Source: CAD feature listing. Evaluate the final solid. Frame: model axes, mm. Round coordinates to 2 decimals unless told otherwise and drop trailing zeros. Loops run counter-clockwise (first coordinate to the right, second up) from the corner with the lowest first, then second, coordinate; pieces in that order, holes last. Notation, with made-up numbers: (56, 39) - (91, 39) arc R13 ccw to (91, 45) - close; hole circle Ø11 at (15, 20.5). An arc over 180 degrees is marked (long way). One line per question, with ' | ' between items.
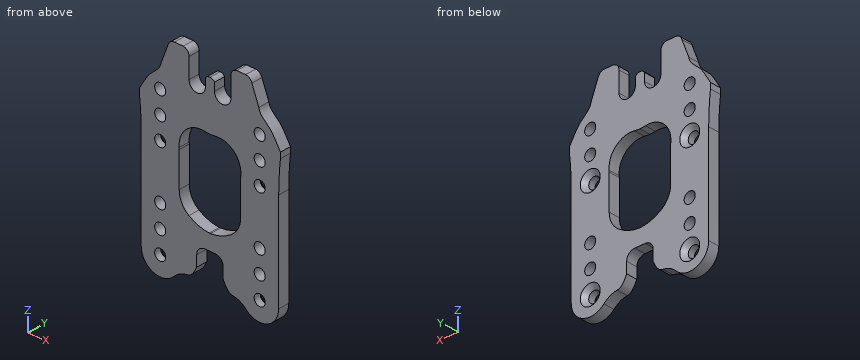
from build123d import *

# Parameters (mm, degrees)
BOSS_EXTRUDE1_DEPTH            = 5
M6_CLEARANCE_HOLE1_D           = 5
M6_CLEARANCE_HOLE1_CSINK_D     = 9
M6_CLEARANCE_HOLE1_CSINK_ANGLE = 90
M6X1_0_TAPPED_HOLE1_D          = 5


with BuildPart() as part:
    # Sketch1 → Boss-Extrude1 (new body)
    with BuildSketch(Plane(origin=(0, 0, 0), x_dir=(1, 0, 0), z_dir=(0, 1, 0))):
        with BuildLine():
            Line((69.154429566, 13.47085249), (69.154429566, 16.004009211))
            ThreePointArc((69.154429566, 16.004009211), (68.568623983, 23.140876552), (68.373161278, 30.2990773))
            Line((68.373161278, 30.2990773), (68.373161278, 48.133269951))
            Line((68.373161278, 48.133269951), (68.373161278, 53.582502285))
            Line((68.373161278, 53.582502285), (68.373161278, 74.2990773))
            ThreePointArc((68.373161278, 74.2990773), (63.00118115, 82.261470023), (53.60664117, 80.261348294))
            ThreePointArc((53.60664117, 80.261348294), (50.863204763, 78.250955414), (47.60463673, 77.276349225))
            add(Edge.make_bspline(
                [(43.284305461, 72.691623988), (43.987930263, 74.072264243), (45.137867804, 76.695348328), (47.258032118, 77.234650193), (47.60463673, 77.276349225)],
                knots=[0, 0, 0, 0, 0.393067042, 0.466810905, 0.466810905, 0.466810905, 0.466810905], degree=3))
            Line((43.284305461, 72.691623988), (43.284305461, 67.837570304))
            ThreePointArc((43.284305461, 67.837570304), (42.213675848, 65.252841772), (39.628947316, 64.182212159))
            Line((39.628947316, 64.182212159), (34.94347173, 64.182212159))
            ThreePointArc((34.94347173, 64.182212159), (32.358743198, 65.252841772), (31.288113585, 67.837570304))
            Line((31.288113585, 67.837570304), (31.288113585, 72.691623988))
            add(Edge.make_bspline(
                [(31.288113585, 72.691623988), (30.584488782, 74.072264242), (29.434551241, 76.695348328), (27.314386927, 77.234650193), (26.967782316, 77.276349225)],
                knots=[0, 0, 0, 0, 0.393067042, 0.466810905, 0.466810905, 0.466810905, 0.466810905], degree=3))
            ThreePointArc((26.967782316, 77.276349225), (23.709214283, 78.250955414), (20.965777876, 80.261348294))
            ThreePointArc((20.965777876, 80.261348294), (11.571237896, 82.261470023), (6.199257768, 74.2990773))
            Line((6.199257768, 74.2990773), (6.199257768, 53.582502285))
            Line((6.199257768, 53.582502285), (6.199257768, 48.133269951))
            Line((6.199257768, 48.133269951), (6.199257768, 30.2990773))
            ThreePointArc((6.199257768, 30.2990773), (6.003795063, 23.140876552), (5.41798948, 16.004009211))
            Line((5.41798948, 16.004009211), (5.41798948, 13.47085249))
            add(Edge.make_bspline(
                [(5.41798948, 13.47085249), (7.046412561, 10.903861817), (9.447890726, 5.623503132), (14.765538488, 2.695653096), (15.189698257, -0.049535855)],
                knots=[0, 0, 0, 0, 0.546916624, 1, 1, 1, 1], degree=3))
            Line((15.189698257, -0.049535855), (18.315949534, -8.138840351))
            ThreePointArc((18.315949534, -8.138840351), (19.364485683, -9.737903523), (21.173403671, -10.357779963))
            Line((21.173403671, -10.357779963), (25.170614374, -10.357779963))
            ThreePointArc((25.170614374, -10.357779963), (27.074415678, -9.397871639), (27.84130194, -7.408457441))
            Line((27.84130194, -7.408457441), (27.84130194, 1.545841867))
            ThreePointArc((27.84130194, 1.545841867), (31.527431336, 5.231971263), (35.213560733, 1.545841867))
            Line((35.213560733, 1.545841867), (35.213560733, -1.95624117))
            ThreePointArc((35.213560733, -1.95624117), (36.093993872, -2.799009437), (37.286209528, -3.05207602))
            ThreePointArc((37.286209528, -3.05207602), (38.478425184, -2.799009437), (39.358858323, -1.95624117))
            Line((39.358858323, -1.95624117), (39.358858323, 1.545841867))
            ThreePointArc((39.358858323, 1.545841867), (43.044987714, 5.231971258), (46.731117106, 1.545841867))
            Line((46.731117106, 1.545841867), (46.731117106, -7.408457441))
            ThreePointArc((46.731117106, -7.408457441), (47.498003369, -9.39787164), (49.401804673, -10.357779963))
            Line((49.401804673, -10.357779963), (53.399015375, -10.357779963))
            ThreePointArc((53.399015375, -10.357779963), (55.207933362, -9.737903523), (56.256469511, -8.138840351))
            Line((56.256469511, -8.138840351), (59.382720789, -0.049535855))
            add(Edge.make_bspline(
                [(69.154429566, 13.47085249), (67.526006485, 10.903861817), (65.12452832, 5.623503132), (59.806880557, 2.695653096), (59.382720789, -0.049535855)],
                knots=[0, 0, 0, 0, 0.546916624, 1, 1, 1, 1], degree=3))
        make_face()
        with BuildLine():
            Line((37.590365628, 57.198418754), (36.982053418, 57.198418754))
            add(Edge.make_bspline(
                [(27.789822398, 54.075777582), (30.499523282, 55.89941311), (33.552733603, 57.080263172), (36.982053418, 57.198418754)],
                knots=[0.681705089, 0.681705089, 0.681705089, 0.681705089, 1, 1, 1, 1], degree=3))
            ThreePointArc((27.789822398, 54.075777582), (24.546117922, 50.47890197), (23.373161278, 45.779614194))
            Line((23.373161278, 45.779614194), (23.373161278, 30.2990773))
            ThreePointArc((23.373161278, 30.2990773), (23.364804799, 29.920337919), (23.339751629, 29.542335687))
            ThreePointArc((23.339751629, 29.542335687), (26.460419501, 21.366644617), (34.819518268, 18.777057732))
            add(Edge.make_bspline(
                [(34.819518268, 18.777057732), (35.231027882, 18.840286024), (36.0539589, 18.949507928), (36.875794913, 19.003560622), (37.286209523, 19.011619704)],
                knots=[0.850973756, 0.850973756, 0.850973756, 0.850973756, 0.895462137, 0.939950518, 0.939950518, 0.939950518, 0.939950518], degree=3))
            add(Edge.make_bspline(
                [(39.752900778, 18.777057732), (39.341391163, 18.840286024), (38.518460146, 18.949507928), (37.696624133, 19.003560622), (37.286209523, 19.011619704)],
                knots=[0.850973756, 0.850973756, 0.850973756, 0.850973756, 0.895462137, 0.939950518, 0.939950518, 0.939950518, 0.939950518], degree=3))
            ThreePointArc((39.752900778, 18.777057732), (48.111999545, 21.366644617), (51.232667416, 29.542335687))
            ThreePointArc((51.232667416, 29.542335687), (51.207614246, 29.920337919), (51.199257768, 30.2990773))
            Line((51.199257768, 30.2990773), (51.199257768, 45.779614194))
            ThreePointArc((51.199257768, 45.779614194), (50.026301124, 50.47890197), (46.782596648, 54.075777582))
            add(Edge.make_bspline(
                [(46.782596648, 54.075777582), (44.072895763, 55.89941311), (41.019685443, 57.080263172), (37.590365628, 57.198418754)],
                knots=[0.681705089, 0.681705089, 0.681705089, 0.681705089, 1, 1, 1, 1], degree=3))
        make_face(mode=Mode.SUBTRACT)
    extrude(amount=BOSS_EXTRUDE1_DEPTH)

    # M6 Clearance Hole1 (through all)
    with Locations(Plane(origin=(0, 5, 0), x_dir=(1, 0, 0), z_dir=(0, 1, 0))):
        with Locations((14.786209523, 74.2990773), (59.786209523, 74.2990773), (14.786209523, 30.2990773), (59.786209523, 30.2990773)):
            CounterSinkHole(M6_CLEARANCE_HOLE1_D / 2, M6_CLEARANCE_HOLE1_CSINK_D / 2, counter_sink_angle=M6_CLEARANCE_HOLE1_CSINK_ANGLE)

    # M6x1.0 Tapped Hole1 (through all)
    with Locations(Plane(origin=(0, 5, 0), x_dir=(1, 0, 0), z_dir=(0, 1, 0))):
        with Locations((14.786209523, 54.2990773), (59.786209523, 54.2990773), (14.786209523, 10.2990773), (59.786209523, 10.2990773), (14.786209523, 64.2990773), (59.786209523, 64.2990773), (59.786209523, 20.2990773), (14.786209523, 20.2990773)):
            Hole(M6X1_0_TAPPED_HOLE1_D / 2)


solid = part.part
1. Section query C-C, the plane z = -60.5. Return loops of the section in (x, y), plus the area to 3 significant figures.
Worked out:
outline: (6.2, 0) - (68.37, 0) - (68.37, 5) - (6.2, 5) - close | area: 311 mm2
2. Section query A-A, the plane z = -37. Return loops of the section in (x, y).
Worked out:
outline: (6.2, 0) - (23.37, 0) - (23.37, 5) - (6.2, 5) - close; (51.2, 0) - (68.37, 0) - (68.37, 5) - (51.2, 5) - close
3. Material intervals for probe 1 along X at (y, z) = (4.7, -31.5); probe 2 along X at (y, z) = (0.4, -12); probe 3 along X at (y, z) = (1.85, -68.5), sorted ascending.
Worked out:
probe 1: x = 6.2 to 10.76, 18.81 to 23.37, 51.2 to 55.76, 63.81 to 68.37 | probe 2: x = 6.31 to 12.95, 16.62 to 57.95, 61.62 to 68.26 | probe 3: x = 6.2 to 31.29, 43.28 to 68.37
4. Contact query for flat-ended pins moving along their axis: P1, Ø1.5, axis at y = 1.5, z = -53, coming from the +X side; P2, Ø1.8, axis at y = 2, z = -0.5, coming from the +X side; P3, Ø2.5, axis at y = 1.5, z = 2, coming from the +X side. Output: stop coordinate, or through.
Worked out:
P1: stops at x = 68.37 | P2: stops at x = 59.83 | P3: stops at x = 59.11
5. Section query B-B, the plane y = 1.25. Give the number of separate pieces and of enclosed holes in the cut face, plus the area to 3 significant figures.
Worked out:
separate pieces: 1 | enclosed holes: 13 | area: 3,650 mm2
